Work out the finished part from the listing and answer in its coordinate system (mm). Face numbers are marked on the shaded views. Coordinates: 2 decimals unless noted, no trailing zeros. Order: outer loops, then holes, each group sorted by start corner. A loop starts at its lowest first (then second) coordinate and runs counter-clockwise, first axis right, second up. Notation, with made-up numbers: M 60,-28 L 115,-28 A26 ccw 115,9 Z; hole C 84,47 d5. An arc over 180 degrees is marked long. Write item = value, one per line. Start each with the question number.
Q1. Find section C-C on z = 2.8. Give the vertices of the cut face in (x, y), and give its area (3 significant figures).
Q2. Straight lines are drawn through the part: line 1 along Y through (x, z) = (30, 3.25); line 2 along X through (y, z) = (3.25, 2.6); line 3 along X through (y, z) = (-3.5, 0.7). For each, find the intervals that lie inside material, in ascending order.
Q3. Determine the mould class of the marked faces 1, 2, 3 and 4 for opening direction Y: released by +Y, released by -Y, zero draft, split by the parting line, or undercut.
Q4. Find section A-A on x = 30. Give the vertices of the cut face in (y, z).
Q5. Find section D-D on y = -2.75. Give the vertices of the cut face in (x, z).
Q6. Each of these flat-tipped pins is pushed along its axis until it touches: P1, Ø1.5, axis at x = 17, y = 2, coming from the -Z side; P2, Ø9, axis at x = 30, y = 0, coming from the +Z side. Where does it stop, or does it pass through?
Q7. Find section B-B on y = 0. Give the vertices of the cut face in (x, z).
```python
from build123d import *

# Parameters (mm, degrees)
F0_W     = 50
F0_H     = 20
F1_DEPTH = 5
F2_R     = 5
F3_DEPTH = 5
F4_R     = 5
F5_DEPTH = 5
F6_R     = 5


with BuildPart() as f1:
    # F0 (on Top) → F1 (new body)
    with BuildSketch(Plane.XY):
        with Locations((15, 0)):
            Rectangle(F0_W, F0_H)
    extrude(amount=F1_DEPTH)

    # F2 (on face) → F3 (cut, through all)
    with BuildSketch(Plane.XY.offset(5)):
        Circle(F2_R)
    extrude(amount=-F3_DEPTH, mode=Mode.SUBTRACT)

    # F4 (on face) → F5 (cut, through all)
    with BuildSketch(Plane.XY.offset(5)):
        with Locations((30, 0)):
            Circle(F4_R)
    extrude(amount=-F5_DEPTH, mode=Mode.SUBTRACT)

    # F6
    f6_edges = [f1.edges().sort_by_distance(p)[0] for p in [
        (-10, 10, 2.5),
        (-10, -10, 2.5),
        (40, 10, 2.5),
        (40, -10, 2.5),
    ]]
    fillet(f6_edges, radius=F6_R)


solid = f1.part
```
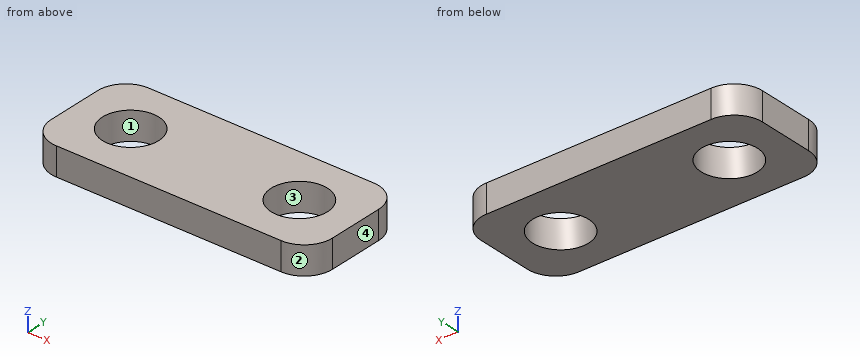
Findings below:
q1.outline = M -10,-5 A5 ccw -5,-10 L 35,-10 A5 ccw 40,-5 L 40,5 A5 ccw 35,10 L -5,10 A5 ccw -10,5 Z; hole C 0,0 d10; hole C 30,0 d10
q1.area = 821 mm^2
q2.line_1 = -10 to -5, 5 to 10
q2.line_2 = -10 to -3.8, 3.8 to 26.2, 33.8 to 40
q2.line_3 = -10 to -3.57, 3.57 to 26.43, 33.57 to 40
q3.face_1 = undercut
q3.face_2 = released by -Y
q3.face_3 = undercut
q3.face_4 = zero draft
q4.outline = M -10,0 L -5,0 L -5,5 L -10,5 Z; M 5,0 L 10,0 L 10,5 L 5,5 Z
q5.outline = M -10,0 L -4.18,0 L -4.18,5 L -10,5 Z; M 4.18,0 L 25.82,0 L 25.82,5 L 4.18,5 Z; M 34.18,0 L 40,0 L 40,5 L 34.18,5 Z
q6.P1 = 0
q6.P2 = through
q7.outline = M -10,0 L -5,0 L -5,5 L -10,5 Z; M 5,0 L 25,0 L 25,5 L 5,5 Z; M 35,0 L 40,0 L 40,5 L 35,5 Z
